Print and shaded views of the part. All mm, measured from the part's lowest x, y and z. A direction names the side the tool comes from. Give positions to 0.01 mm unless a question says otherwise; leave off trailing zeros. Loops run counter-clockwise (first coordinate to the right, second up) from the corner with the lowest first, then second, coordinate; pieces in that order, holes last. Notation, with made-up numbers: M 68,62.25 L 122,62.25 A13 cw 122,67.25 Z; hole C 58.5,42 d5. An arc over 180 degrees is marked long. Answer as CSV lines item,"result".
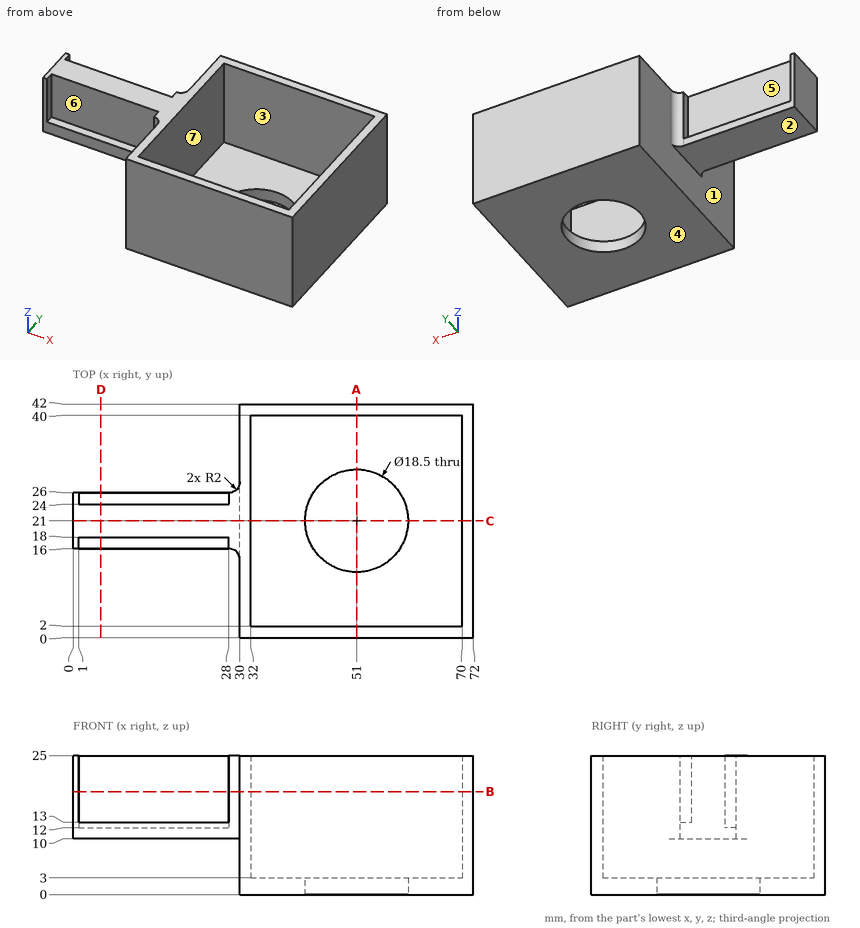
Q1. Cut at B-B (z = 18.5). Write the cut outline in (x, y).
Solution:
outline,"M 0,16 L 1,16 L 1,18 L 28,18 L 28,16 A2 cw 30,14 L 30,0 L 72,0 L 72,42 L 30,42 L 30,28 A2 cw 28,26 L 28,24 L 1,24 L 1,26 L 0,26 Z; hole M 32,2 L 70,2 L 70,40 L 32,40 Z"
Q2. Mould opens along Y. For the marked faces 5, 6 and 7 say: released by +Y, released by -Y, zero draft, split by the parting line, or undercut.
Solution:
face 5,"released by +Y"
face 6,"released by -Y"
face 7,"undercut"
Q3. Pin check, flat tips, straight feed: P1, Ø4.5, axis at x = 19.5, z = 15, coming from the +Y side; P2, Ø10, axis at x = 62, y = 9.5, coming from the +Z side; P3, Ø11, axis at x = 15, y = 20, coming from the -Z side. Stop position of each tip, or through.
Solution:
P1,"stops at y = 24"
P2,"stops at z = 3"
P3,"stops at z = 10"
Q4. Wall check: line 1 (X direction, y = 16.5, z = 20.25); line 2 (X direction, y = 13, z = 12.5); line 3 (Y direction, x = 51, z = 2). Give the ranges that are in metal, low to high. Write a range as [from, to].
Solution:
line 1,"x = [0, 1], [28, 32], [70, 72]"
line 2,"x = [30, 32], [70, 72]"
line 3,"y = [0, 11.75], [30.25, 42]"
Q5. Cut at D-D (x = 5). Write the cut outline in (y, z).
Solution:
outline,"M 16,10 L 26,10 L 26,12 L 24,12 L 24,25 L 18,25 L 18,13 L 16,13 Z"
Q6. Cut at C-C (y = 21). Write the cut outline in (x, z), and give its area (4 significant figures).
Solution:
outline,"M 0,10 L 30,10 L 30,0 L 41.75,0 L 41.75,3 L 32,3 L 32,25 L 0,25 Z; M 60.25,0 L 72,0 L 72,25 L 70,25 L 70,3 L 60.25,3 Z"
area,"608.5 mm²"
Q7. Cut at A-A (x = 51). Write the cut outline in (y, z), and give its area (4 significant figures).
Solution:
outline,"M 0,0 L 11.75,0 L 11.75,3 L 2,3 L 2,25 L 0,25 Z; M 30.25,0 L 42,0 L 42,25 L 40,25 L 40,3 L 30.25,3 Z"
area,"158.5 mm²"
Q8. Which spindle directions (+Z, -Z, +X, -X, +Y, -Y) get a long thin tool onto all of the face, cutting with end or side? Do the marked faces 1, 2, 3 and 4. Say none if no direction does.
Solution:
face 1,"-Z, -X"
face 2,"-Z, -X, +Y, -Y"
face 3,"+Z"
face 4,"-Z, +X, -X, +Y, -Y"
